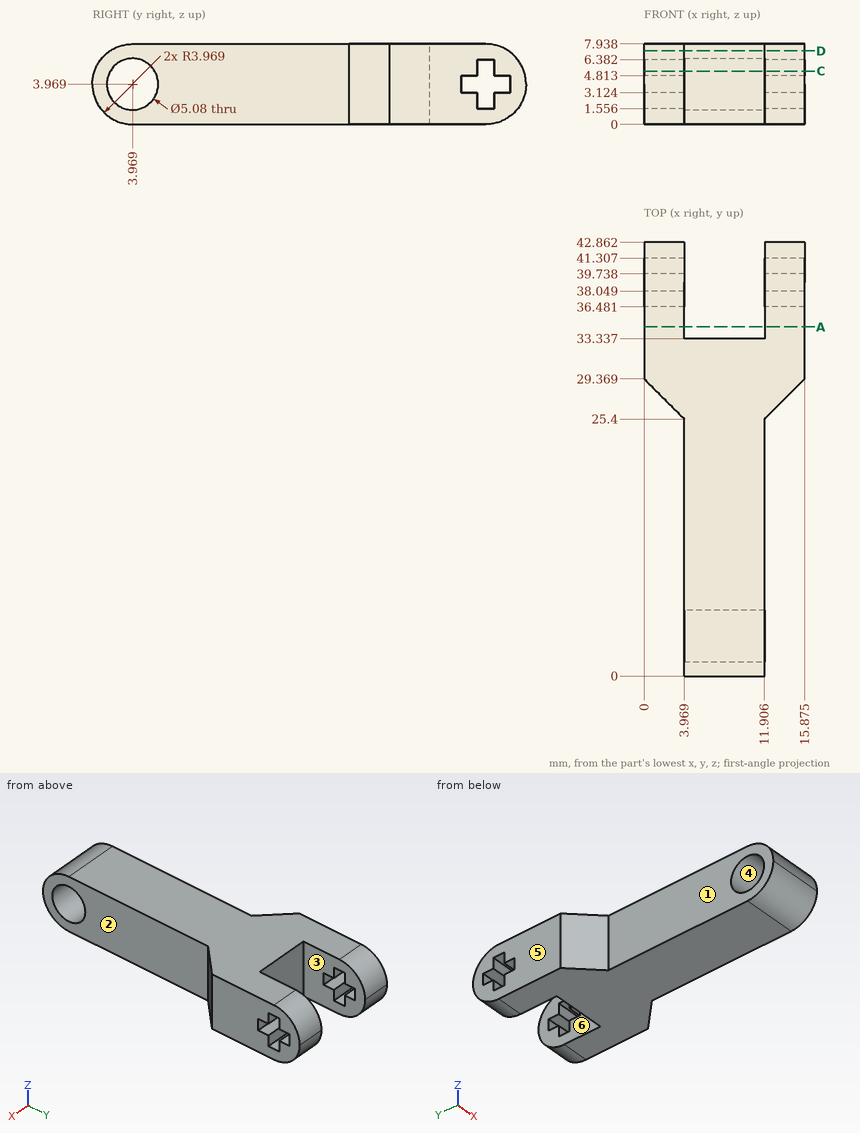
Study the drawing (mm; zero at the part's minimum x, y, z) and answer. A direction names the side the tool comes from. Give positions to 0.01 mm unless a question says otherwise; leave off trailing zeros. Order: outer loops, then holes, each group sorted by start corner. A loop starts at its lowest first (then second) coordinate and runs counter-clockwise, first axis right, second up. Notation, with made-up numbers: (22.25, 1.5) - (66.25, 1.5) arc R16 cw to (66.25, 26.5) - close; hole circle Ø2 at (46.5, 66.5). An arc over 180 degrees is marked (long way). Answer in a Markdown table with one row per item. Add a question column.
Q1. The part is cut by section A-A (y = 34.5). Determine the outline of the cut face in (x, z) (1 decimal).
Q2. For a pull along X with two mould halves and no side action, classify the marked faces 4, 5 and 6 as released by +X, released by -X, zero draft, split by the parting line, or undercut.
Q3. The part is cut by section C-C (z = 5.25). Give the number of separate pieces and of enclosed holes in the cut face, then the cut area to 3 significant figures.
Q4. Given P1, Ø1.3, axis at x = 3, y = 41, coming from the -Z side; P2, Ø2.5, axis at y = 39, z = 5, coming from the -X side; P3, Ø1.3, axis at x = 15, z = 2.5, coming from the -Y side (1 decimal); P4, Ø3, axis at x = 6, z = 6.5, coming from the -Y side, each flat-ended and moving along its own axis, determine where each tip first touches the part or whether it passes through.
Q5. Which of the six approach directions +Z, -Z, +X, -X, +Y, -Y give full straight-line access (tool end or side, diameter ignored) to the marked faces 1, 2 and 3?
Q6. Find the intervals of material crossed by line 1 along X through (y, z) = (37.5, 0.5) (1 decimal); line 2 along X through (y, z) = (20, 3.5); line 3 along Y through (x, z) = (2, 4) (1 decimal), in increasing order. Write a range as [from, to].
Q7. The part is cut by section D-D (z = 7.25). Determine the outline of the cut face in (x, y) (1 decimal).
Determined:
| question | item | result |
|---|---|---|
| 1 | outline | (0, 0) - (4, 0) - (4, 7.9) - (0, 7.9) - close; (11.9, 0) - (15.9, 0) - (15.9, 7.9) - (11.9, 7.9) - close |
| 2 | face 4 | zero draft |
| 2 | face 5 | released by -X |
| 2 | face 6 | undercut |
| 3 | separate pieces | 4 |
| 3 | enclosed holes | 0 |
| 3 | area | 336 mm² |
| 4 | P1 | stops at z = 0.28 |
| 4 | P2 | stops at x = 0 |
| 4 | P3 | stops at y = 27.8 |
| 4 | P4 | stops at y = 0.14 |
| 5 | face 1 | +Z, -Z, -X, -Y |
| 5 | face 2 | +Z, -Z, +X, -Y |
| 5 | face 3 | +Z, -Z, +Y |
| 6 | line 1 | x = [0, 4], [11.9, 15.9] |
| 6 | line 2 | x = [3.97, 11.91] |
| 6 | line 3 | y = [27.4, 36.5], [41.3, 42.9] |
| 7 | outline | (0, 29.4) - (4, 25.4) - (4, 1.7) - (11.9, 1.7) - (11.9, 25.4) - (15.9, 29.4) - (15.9, 41.1) - (11.9, 41.1) - (11.9, 33.3) - (4, 33.3) - (4, 41.1) - (0, 41.1) - close |
